Here's how the part is built. I have some questions about the finished solid (model axes, mm). Face numbers are marked on the shaded views. A direction names the side the tool comes from. Give positions to 0.01 mm unless a question says otherwise; leave off trailing zeros. Loops run counter-clockwise (first coordinate to the right, second up) from the corner with the lowest first, then second, coordinate; pieces in that order, holes last.
Q1. Suppose I cut it at A-A (y = 31). List the corners of the cut face in (x, z) for me, and give its area (3 significant figures).
Q2. For the marked faces 1, 2 and 3, which set-ups out of +Z, -Z, +X, -X, +Y, -Y let a thin tool reach every point of the face, with its end or its side?
Q3. Suppose I cut it at B-B (z = -1.5). List the corners of the cut face in (x, y) for me.
Q4. Suppose I cut it at C-C (z = 0.5). List the corners of the cut face in (x, y) for me, and give its area (3 significant figures).
Q5. I need wall thicknesses on probe 1 along Z at (x, y) = (-26, 18.5); probe 2 along Y at (x, z) = (-35.5, -1.5); probe 3 along Y at (x, z) = (-35.5, -3.25). Which ranges of each line are inside material? Lowest first, please.
Q6. I'm going to push flat-ended pins straight in: P1, Ø3.5, axis at x = -20.22, y = 29.1, coming from the -Z side; P2, Ø3, axis at y = 17.5, z = -3, coming from the -X side; P3, Ø1.3, axis at x = -36, z = -1.5, coming from the +Y side. Where does each tip first touch, or does it pass through?
Q7. Suppose I cut it at D-D (y = 21.25). List the corners of the cut face in (x, z) for me, and give its area (3 significant figures).
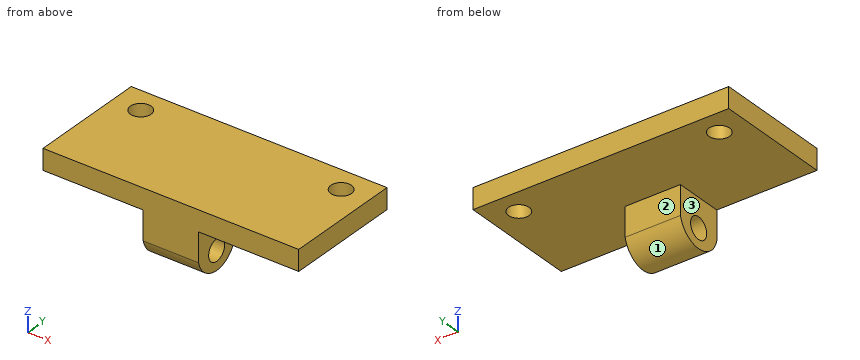
```python
from build123d import *

# Parameters (mm, degrees)
CROQUIS1_W              = 37
CROQUIS1_H              = 13
SALIENTE_EXTRUIR1_DEPTH = 3
CROQUIS3_W              = 8
CROQUIS3_H              = 7
SALIENTE_EXTRUIR2_DEPTH = 7
CROQUIS6_R              = 1.55
CORTAR_EXTRUIR4_DEPTH   = 8
CROQUIS8_W              = 37
CROQUIS8_H              = 3
SALIENTE_EXTRUIR3_DEPTH = 4
CROQUIS9_R              = 1.5
CORTAR_EXTRUIR5_DEPTH   = 3


with BuildPart() as part:
    # Croquis1 → Saliente-Extruir1 (new body)
    with BuildSketch(Plane.XY):
        with Locations((-34.723076923, 22.103846154)):
            Rectangle(CROQUIS1_W, CROQUIS1_H)
    extrude(amount=SALIENTE_EXTRUIR1_DEPTH)

    # Croquis3 → Saliente-Extruir2 (add)
    with BuildSketch(Plane(origin=(0, 0, 0), x_dir=(-1, 0, 0), z_dir=(0, 0, -1))):
        with Locations((34.723076923, 19.103846154)):
            Rectangle(CROQUIS3_W, CROQUIS3_H)
    extrude(amount=SALIENTE_EXTRUIR2_DEPTH)

    # Croquis6 → Cortar-Extruir4 (cut)
    with BuildSketch(Plane(origin=(-30.723076923, 0, 0), x_dir=(0, 0, -1), z_dir=(1, 0, 0))):
        with Locations((4.200477656, 19.103846154)):
            Circle(CROQUIS6_R)
        with BuildLine():
            Line((4.200477656, 22.603846154), (7, 22.603846154))
            Line((7, 22.603846154), (7, 15.603846154))
            Line((7, 15.603846154), (4.200477656, 15.603846154))
            ThreePointArc((4.200477656, 15.603846154), (6.987743364, 19.103846154), (4.200477656, 22.603846154))
        make_face()
    extrude(amount=-CORTAR_EXTRUIR4_DEPTH, mode=Mode.SUBTRACT)

    # Croquis8 → Saliente-Extruir3 (add)
    with BuildSketch(Plane(origin=(0, 28.603846154, 0), x_dir=(1, 0, 0), z_dir=(0, 1, 0))):
        with Locations((-34.723076923, -1.5)):
            Rectangle(CROQUIS8_W, CROQUIS8_H)
    extrude(amount=SALIENTE_EXTRUIR3_DEPTH)

    # Croquis9 → Cortar-Extruir5 (cut)
    with BuildSketch(Plane(origin=(0, 0, 0), x_dir=(-1, 0, 0), z_dir=(0, 0, -1))):
        with Locations((20.223076923, 29.103846154)):
            Circle(CROQUIS9_R)
        with Locations((49.223076923, 29.103846154)):
            Circle(CROQUIS9_R)
    extrude(amount=-CORTAR_EXTRUIR5_DEPTH, mode=Mode.SUBTRACT)


solid = part.part
```
Solutions:
1. outline: (-53.22, 0) - (-16.22, 0) - (-16.22, 3) - (-53.22, 3) - close
1. area: 111 mm2
2. face 1: -Z, +X, -X
2. face 2: -Z, +X, -X, +Y
2. face 3: -Z, -X, +Y, -Y
3. outline: (-38.72, 15.6) - (-30.72, 15.6) - (-30.72, 22.6) - (-38.72, 22.6) - close
4. outline: (-53.22, 15.6) - (-16.22, 15.6) - (-16.22, 32.6) - (-53.22, 32.6) - close; hole circle Ø3 at (-49.22, 29.1); hole circle Ø3 at (-20.22, 29.1)
4. area: 615 mm2
5. probe 1: z = 0 to 3
5. probe 2: y = 15.6 to 22.6
5. probe 3: y = 15.6 to 17.88, 20.33 to 22.6
6. P1: stops at z = 0
6. P2: stops at x = -38.72
6. P3: stops at y = 22.6
7. outline: (-53.22, 0) - (-38.72, 0) - (-38.72, -6.28) - (-30.72, -6.28) - (-30.72, 0) - (-16.22, 0) - (-16.22, 3) - (-53.22, 3) - close
7. area: 161 mm2
